Input: dimensioned drawing with shaded views. Units: mm. Origin: part minimum x, y, z. Round coordinates to 2 decimals unless told otherwise and drop trailing zeros. Loops run counter-clockwise (first coordinate to the right, second up) from the corner with the lowest first, then second, coordinate; pieces in that order, holes last. Notation, with made-up numbers: M -8.75,30.5 L 13.25,30.5 A4 ccw 13.25,34.5 Z; hole C 58.25,89 d9. An arc over 180 degrees is marked long. One line per item, written item: value.
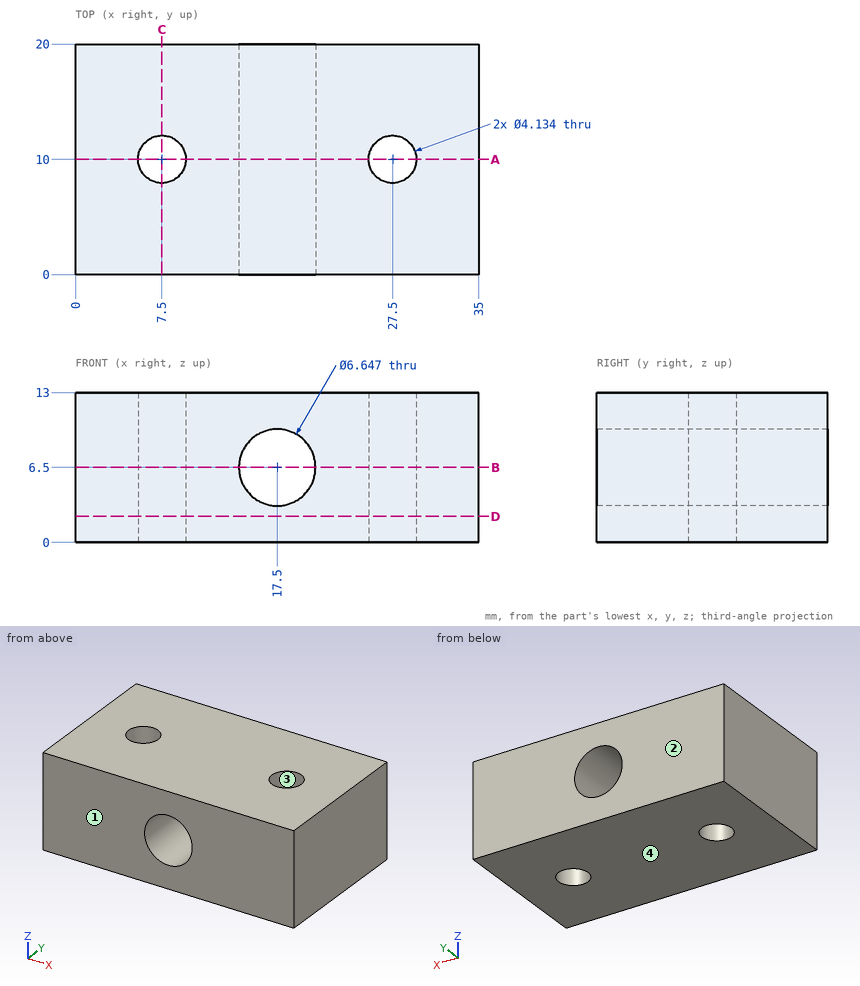
1. Section query B-B (z = 6.5). Return the cut outline in (x, y).
Report:
outline: M 0,0 L 14.18,0 L 14.18,20 L 0,20 Z; M 20.82,0 L 35,0 L 35,20 L 20.82,20 Z; hole C 7.5,10 d4.13; hole C 27.5,10 d4.13
2. Pull-direction query (Y, two-part tool) for the marked faces 1, 2, 3 and 4; classes: released by +Y, released by -Y, zero draft, split by the parting line, or undercut.
Report:
face 1: released by -Y
face 2: released by +Y
face 3: undercut
face 4: zero draft
3. Section query A-A (y = 10). Return the cut outline in (x, z).
Report:
outline: M 0,0 L 5.43,0 L 5.43,13 L 0,13 Z; M 9.57,0 L 25.43,0 L 25.43,13 L 9.57,13 Z; M 29.57,0 L 35,0 L 35,13 L 29.57,13 Z; hole C 17.5,6.5 d6.65
4. Ray query, line 1 (X direction, y = 10, z = 3); line 2 (Y direction, x = 7.5, z = 5); line 3 (X direction, y = 9, z = 1.5). Return the intervals inside material, ascending. Write a range as [from, to].
Report:
line 1: x = [0, 5.43], [9.57, 25.43], [29.57, 35]
line 2: y = [0, 7.93], [12.07, 20]
line 3: x = [0, 5.69], [9.31, 25.69], [29.31, 35]
5. Section query C-C (x = 7.5). Return the cut outline in (y, z).
Report:
outline: M 0,0 L 7.93,0 L 7.93,13 L 0,13 Z; M 12.07,0 L 20,0 L 20,13 L 12.07,13 Z
6. Section query D-D (z = 2.25). Return the cut outline in (x, y).
Report:
outline: M 0,0 L 35,0 L 35,20 L 0,20 Z; hole C 7.5,10 d4.13; hole C 27.5,10 d4.13
7. Pin query (flat end, axial travel): pin 1 (5.5 mm diameter, centred on x = 17.5, z = 6.5, fed in from +Y). Return the tip coordinate at first contact, or that it passes through.
Report:
pin 1: passes through
